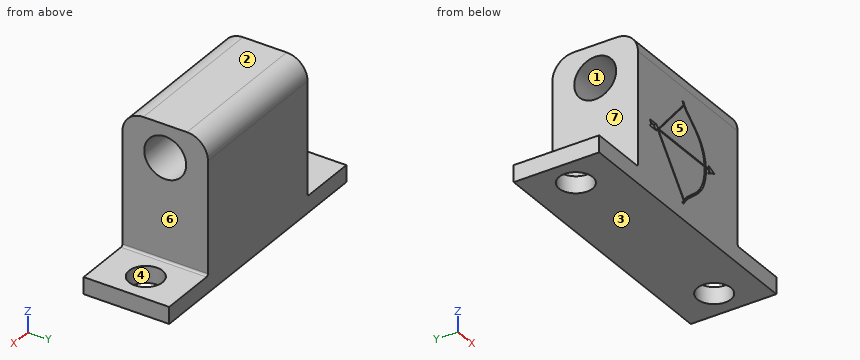
Autodesk Fusion 360 part; units mm, degrees
sketch "Sketch1" plane through (0, 0, 0) normal (0, 0, 1) x (1, 0, 0)
  line L0 (0, 0) -> (32, 0)
  line L1 (32, 0) -> (32, 10.2)
  line L2 (32, 10.2) -> (0, 10.2)
  line L3 (0, 10.2) -> (0, 0)
  dimension "d1" = 32
  dimension "d2" = 10.2
extrude "Extrude1" add sketch "Sketch1" along normal blind 2
sketch "Sketch2" plane through (0, 0, 2) normal (0, 0, 1) x (-1, 0, 0)
  line L0 (0, -10.2) -> (0, 0)
  line L1 (0, 0) -> (-32, 0)
  line L2 (-32, 0) -> (-32, -10.2)
  line L3 (-32, -10.2) -> (0, -10.2)
  line L4 (-7, -10.2) -> (-25, -10.2)
  line L5 (-25, -10.2) -> (-25, 0)
  line L6 (-25, 0) -> (-7, 0)
  line L7 (-7, 0) -> (-7, -10.2)
  circle A0 centre (-3.5, -5.1) radius 2
  circle A1 centre (-28.5, -5.1) radius 2
  dimension "d5" = 7
  dimension "d6" = 7
  dimension "d7" = 5.1
  dimension "d8" = 3.5
  dimension "d9" = 4
  dimension "d10" = 3.5
  dimension "d11" = 5.1
  dimension "d12" = 4
extrude "Extrude2" cut sketch "Sketch2" against normal blind 2.1 contours A0 | A1
extrude "Extrude3" add sketch "Sketch2" along normal blind 16 contours L1 L3 L4 L5 L6 L7
sketch "Sketch3" plane through (25, 0, 0) normal (1, 0, 0) x (0, 1, 0)
  line L0 (0, 2) -> (10.2, 2)
  line L1 (10.2, 2) -> (10.2, 18)
  line L2 (10.2, 18) -> (0, 18)
  line L3 (0, 18) -> (0, 2)
  circle A0 centre (5.1, 14.1) radius 2.5
  dimension "d17" = 3.9
  dimension "d18" = 5.1
  dimension "d19" = 5
extrude "Extrude4" cut sketch "Sketch3" against normal blind 20 contours A0
fillet "Fillet1" radius 2.5 2 edges at (16, 0, 18) (16, 10.2, 18)
fillet "Fillet2" radius 0.25 2 edges at (25, 5.1, 2) (7, 5.1, 2)
sketch "Sketch4" plane through (0, 0, 0) normal (0, -1, 0) x (1, 0, 0)
  line L0 (25, 15.5) -> (7, 15.5)
  line L1 (7, 15.5) -> (7, 2.25)
  arc A0 (6.75, 2) -> (7, 2.25) centre (6.75, 2.25) ccw
  line L2 (6.75, 2) -> (0, 2)
  line L3 (0, 2) -> (0, 0)
  line L4 (0, 0) -> (32, 0)
  line L5 (32, 0) -> (32, 2)
  line L6 (32, 2) -> (25.25, 2)
  arc A1 (25, 2.25) -> (25.25, 2) centre (25.25, 2.25) ccw
  line L7 (25, 2.25) -> (25, 15.5)
  line L8 (15.0115, 13.8918) -> (15.2499, 13.8388)
  line L9 (15.0115, 1.9217) -> (15.2499, 1.8688)
  line L10 (15.2499, 2.3085) -> (10.5625, 8.1981)
  line L11 (10.6841, 8.3354) -> (15.2499, 13.4918)
  line L12 (10.817, 8.3354) -> (15.3124, 13.4128)
  line L13 (15.3132, 2.3954) -> (10.6954, 8.1981)
  spline S0 degree 5 poles (15.0115, 13.8918) (15.0366, 13.8331) (15.0755, 13.7537) (15.1214, 13.6739) (15.1743, 13.5935) (15.2341, 13.5126) (15.2499, 13.4918) knots 0 0 0 0 0 0 0.04 0.053771 0.053771 0.053771 0.053771 0.053771 0.053771
  line L14 (15.2177, 13.5342) -> (15.2821, 13.4495)
  spline S1 degree 5 poles (15.2499, 2.3085) (15.2476, 2.3054) (15.194, 2.2294) (15.1434, 2.1527) (15.0959, 2.0753) (15.0514, 1.9972) (15.0115, 1.9217) knots 0.958261 0.958261 0.958261 0.958261 0.958261 0.958261 0.96 1 1 1 1 1 1
  line L15 (15.2777, 2.3478) -> (15.2221, 2.2693)
  line L16 (19.8903, 8.1981) -> (19.6849, 7.759)
  line L17 (19.6849, 7.759) -> (20.8035, 8.2887)
  line L18 (20.8035, 8.2887) -> (19.6849, 8.7197)
  line L19 (19.6849, 8.7197) -> (19.8674, 8.3354)
  spline S2 degree 5 poles (15.2499, 13.8388) (15.275, 13.7801) (15.3328, 13.6621) (15.4428, 13.4833) (15.636, 13.2415) (15.9534, 12.9319) (16.3409, 12.6103) (16.7857, 12.2676) (17.2659, 11.8886) (17.7534, 11.4561) (18.2174, 10.9546) (18.6276, 10.3741) (18.9469, 9.734) (19.126, 9.1768) (19.2132, 8.7476) (19.2502, 8.4653) (19.263, 8.3354) knots 0 0 0 0 0 0 0.04 0.08 0.12 0.16 0.2 0.24 0.28 0.32 0.36 0.4 0.44 0.473865 0.473865 0.473865 0.473865 0.473865 0.473865
  line L20 (19.1848, 9.1287) -> (19.3411, 7.542)
  spline S3 degree 5 poles (19.2746, 8.1981) (19.2853, 8.0482) (19.2958, 7.7438) (19.2774, 7.2862) (19.1846, 6.69) (18.9625, 5.9984) (18.6463, 5.3801) (18.2572, 4.8452) (17.8198, 4.3863) (17.3603, 3.9873) (16.904, 3.6275) (16.4734, 3.2862) (16.0845, 2.9471) (15.7463, 2.6009) (15.5197, 2.3146) (15.375, 2.094) (15.2897, 1.9443) (15.2499, 1.8688) knots 0.481014 0.481014 0.481014 0.481014 0.481014 0.481014 0.52 0.56 0.6 0.64 0.68 0.72 0.76 0.8 0.84 0.88 0.92 0.96 1 1 1 1 1 1
  line L21 (19.2097, 9.1087) -> (19.3396, 7.2875)
  spline S4 degree 5 poles (15.3124, 13.4128) (15.332, 13.3889) (15.4036, 13.3041) (15.5393, 13.1573) (15.762, 12.9459) (16.1025, 12.6633) (16.5474, 12.3206) (17.0276, 11.9416) (17.515, 11.5091) (17.979, 11.0075) (18.3892, 10.427) (18.7131, 9.7778) (18.894, 9.2098) (18.9811, 8.7693) (19.0172, 8.476) (19.0296, 8.3354) knots 0.064218 0.064218 0.064218 0.064218 0.064218 0.064218 0.08 0.12 0.16 0.2 0.24 0.28 0.32 0.36 0.4 0.44 0.476625 0.476625 0.476625 0.476625 0.476625 0.476625
  line L22 (14.9219, 13.8881) -> (15.7028, 12.9376)
  line L23 (18.9651, 9.0672) -> (19.094, 7.6035)
  spline S5 degree 5 poles (19.0398, 8.1981) (19.0483, 8.0587) (19.0561, 7.765) (19.0358, 7.3185) (18.9432, 6.7334) (18.7242, 6.0513) (18.408, 5.433) (18.0189, 4.8982) (17.5814, 4.4393) (17.1219, 4.0403) (16.6657, 3.6805) (16.235, 3.3392) (15.8681, 3.0192) (15.6141, 2.7622) (15.4485, 2.5703) (15.3521, 2.4471) (15.3132, 2.3954) knots 0.483768 0.483768 0.483768 0.483768 0.483768 0.483768 0.52 0.56 0.6 0.64 0.68 0.72 0.76 0.8 0.84 0.88 0.92 0.948678 0.948678 0.948678 0.948678 0.948678 0.948678
  line L24 (18.989, 9.0312) -> (19.0905, 7.3649)
  line L25 (15.7537, 2.9821) -> (14.8727, 1.8087)
  line L26 (10.6954, 8.1981) -> (19.0398, 8.1981)
  line L27 (19.2746, 8.1981) -> (19.8903, 8.1981)
  line L28 (19.263, 8.3354) -> (19.8674, 8.3354)
  line L29 (10.6725, 8.3354) -> (10.3002, 8.665)
  line L30 (10.3002, 8.665) -> (9.1473, 8.665)
  line L31 (9.1473, 8.665) -> (9.409, 8.2777)
  line L32 (9.409, 8.2777) -> (9.1615, 7.917)
  line L33 (9.1615, 7.917) -> (10.3, 7.917)
  line L34 (10.3, 7.917) -> (10.5625, 8.1981)
  line L35 (10.6725, 8.3354) -> (10.6841, 8.3354)
  line L36 (10.817, 8.3354) -> (19.0296, 8.3354)
  point P0 (16.3357, 12.6206)
  point P1 (16.627, 3.4048)
  point P2 (18.7456, 10.1048)
  point P3 (18.825, 5.7617)
  point P4 (18.5867, 5.8147)
  point P5 (18.5072, 10.1578)
  point P6 (16.0973, 12.6736)
  point P7 (16.3886, 3.4577)
extrude "Extrude5" cut sketch "Sketch4" against normal blind 0.3 contours L8 L9 S0 L14 S1 L15 S2 L20 S3 L21 S4 L22 L23 S5 L24 L25 | L16 L17 L18 L19 L20 L21 L27 L28 | L10 L11 L12 L13 L14 L15 L22 L23 L24 L25 L26 L29 L30 L31 L32 L33 L34 L35 L36
sketch "Sketch5" plane through (0, 0, 18) normal (0, 0, 1) x (-1, 0, 0)
  line L0 (-25, -7.7) -> (-7, -7.7)
  line L1 (-7, -7.7) -> (-7, -2.5)
  line L2 (-7, -2.5) -> (-25, -2.5)
  line L3 (-25, -2.5) -> (-25, -7.7)
  line L4 (-7, -10.2) -> (-25, -10.2)
  line L5 (-25, -10.2) -> (-25, 0)
  line L6 (-25, 0) -> (-7, 0)
  line L7 (-7, 0) -> (-7, -10.2)
  point P0 (-7, -10.2)
  point P1 (-25, 0)
sketch "Sketch6" plane through (16, 5.1, 19.1) normal (0, 0, 1) x (1, 0, 0)
  line L0 (-9, 5.1) -> (9, 5.1)
  line L1 (9, 5.1) -> (9, -5.1)
  line L2 (9, -5.1) -> (-9, -5.1)
  line L3 (-9, -5.1) -> (-9, 5.1)
  point P0 (-9, 5.1)
  point P1 (9, -5.1)
extrude "Extrude6" add 1 faces at (19, 4.2333, 18) along direction (0, 0, 1) blind 1.1
sketch "Sketch7" plane through (16, 0, 18.55) normal (0, -1, 0) x (1, 0, 0)
  line L0 (-9, -3.05) -> (9, -3.05)
  line L1 (9, -3.05) -> (9, 0.55)
  line L2 (9, 0.55) -> (-9, 0.55)
  line L3 (-9, 0.55) -> (-9, -3.05)
  point P0 (-9, -3.05)
  point P1 (9, 0.55)
sketch "Sketch8" plane through (0, 0, 0) normal (0, -1, 0) x (1, 0, 0)
  line L0 (9.409, 8.2777) -> (9.1473, 8.665)
  line L1 (9.1473, 8.665) -> (10.3002, 8.665)
  line L2 (10.3002, 8.665) -> (10.6725, 8.3354)
  line L3 (10.6725, 8.3354) -> (10.6841, 8.3354)
  line L4 (10.6841, 8.3354) -> (15.2499, 13.4918)
  spline S0 degree 5 poles (15.2499, 13.4918) (15.2341, 13.5126) (15.1743, 13.5935) (15.1214, 13.6739) (15.0755, 13.7537) (15.0366, 13.8331) (15.0115, 13.8918) knots -0.053771 -0.053771 -0.053771 -0.053771 -0.053771 -0.053771 -0.04 0 0 0 0 0 0
  line L5 (15.0115, 13.8918) -> (15.2499, 13.8388)
  spline S1 degree 5 poles (15.2499, 13.8388) (15.275, 13.7801) (15.3328, 13.6621) (15.4428, 13.4833) (15.636, 13.2415) (15.9534, 12.9319) (16.3409, 12.6103) (16.7857, 12.2676) (17.2659, 11.8886) (17.7534, 11.4561) (18.2174, 10.9546) (18.6276, 10.3741) (18.9469, 9.734) (19.126, 9.1768) (19.2132, 8.7476) (19.2502, 8.4653) (19.263, 8.3354) knots 0 0 0 0 0 0 0.04 0.08 0.12 0.16 0.2 0.24 0.28 0.32 0.36 0.4 0.44 0.473865 0.473865 0.473865 0.473865 0.473865 0.473865
  line L6 (19.263, 8.3354) -> (19.8674, 8.3354)
  line L7 (19.8674, 8.3354) -> (19.6849, 8.7197)
  line L8 (19.6849, 8.7197) -> (20.8035, 8.2887)
  line L9 (20.8035, 8.2887) -> (19.6849, 7.759)
  line L10 (19.6849, 7.759) -> (19.8903, 8.1981)
  line L11 (19.8903, 8.1981) -> (19.2746, 8.1981)
  spline S2 degree 5 poles (19.2746, 8.1981) (19.2853, 8.0482) (19.2958, 7.7438) (19.2774, 7.2862) (19.1846, 6.69) (18.9625, 5.9984) (18.6463, 5.3801) (18.2572, 4.8452) (17.8198, 4.3863) (17.3603, 3.9873) (16.904, 3.6275) (16.4734, 3.2862) (16.0845, 2.9471) (15.7463, 2.6009) (15.5197, 2.3146) (15.375, 2.094) (15.2897, 1.9443) (15.2499, 1.8688) knots 0.481014 0.481014 0.481014 0.481014 0.481014 0.481014 0.52 0.56 0.6 0.64 0.68 0.72 0.76 0.8 0.84 0.88 0.92 0.96 1 1 1 1 1 1
  line L12 (15.2499, 1.8688) -> (15.0115, 1.9217)
  spline S3 degree 5 poles (15.0115, 1.9217) (15.0514, 1.9972) (15.0959, 2.0753) (15.1434, 2.1527) (15.194, 2.2294) (15.2476, 2.3054) (15.2499, 2.3085) knots -1 -1 -1 -1 -1 -1 -0.96 -0.958261 -0.958261 -0.958261 -0.958261 -0.958261 -0.958261
  line L13 (15.2499, 2.3085) -> (10.5625, 8.1981)
  line L14 (10.5625, 8.1981) -> (10.3, 7.917)
  line L15 (10.3, 7.917) -> (9.1615, 7.917)
  line L16 (9.1615, 7.917) -> (9.409, 8.2777)
  line L17 (25, 15.5) -> (7, 15.5)
  line L18 (7, 15.5) -> (7, 2.25)
  arc A0 (6.75, 2) -> (7, 2.25) centre (6.75, 2.25) ccw
  line L19 (6.75, 2) -> (0, 2)
  line L20 (0, 2) -> (0, 0)
  line L21 (0, 0) -> (32, 0)
  line L22 (32, 0) -> (32, 2)
  line L23 (32, 2) -> (25.25, 2)
  arc A1 (25, 2.25) -> (25.25, 2) centre (25.25, 2.25) ccw
  line L24 (25, 2.25) -> (25, 15.5)
  line L25 (7, 15.5) -> (25, 15.5)
  line L26 (25, 15.5) -> (25, 19.1)
  line L27 (25, 19.1) -> (7, 19.1)
  line L28 (7, 19.1) -> (7, 15.5)
  point P0 (25, 19.1)
sketch "Sketch9" plane through (0, 0, 0) normal (0, -1, 0) x (1, 0, 0)
sketch "Sketch10" plane through (25, 0, 0) normal (1, 0, 0) x (0, 1, 0)
  line L0 (0, 2.25) -> (10.2, 2.25)
  line L1 (10.2, 2.25) -> (10.2, 15.5)
  arc A0 (10.2, 15.5) -> (7.7, 18) centre (7.7, 15.5) ccw
  line L2 (7.7, 18) -> (7.7, 19.1)
  line L3 (7.7, 19.1) -> (2.5, 19.1)
  line L4 (2.5, 19.1) -> (2.5, 18)
  arc A1 (2.5, 18) -> (0, 15.5) centre (2.5, 15.5) ccw
  line L5 (0, 15.5) -> (0, 2.25)
  circle A2 centre (5.1, 14.1) radius 2.5
  line L6 (0, 19.1) -> (10.2, 19.1)
  line L7 (10.2, 19.1) -> (10.2, 10)
  line L8 (10.2, 10) -> (0, 10)
  line L9 (0, 10) -> (0, 19.1)
  line L10 (10.2, 2) -> (10.2, 18)
  point P0 (0, 19.1)
extrude "Extrude7" cut 1 faces at (19, 4.2333, 19.1) along direction (0, 0, -1) blind 1.1
Could you check a few things on this model? Use its own coordinates, in mm. Face numbers are marked on the shaded views. A direction names the side the tool comes from. Give positions to 0.01 mm unless a question says otherwise; leave off trailing zeros. Loops run counter-clockwise (first coordinate to the right, second up) from the corner with the lowest first, then second, coordinate; pieces in that order, holes last. Notation, with made-up numbers: (7, 47) - (47, 47) arc R18 cw to (47, 75) - close; hole circle Ø7 at (65.5, 32). An arc over 180 degrees is marked (long way). Use one line per item in the form item = value.
1. I want a section at B-B (y = 5.1). Please give me the cut outline in (x, z).
Response values:
outline = (0, 0) - (1.5, 0) - (1.5, 2) - (0, 2) - close; (5.5, 0) - (26.5, 0) - (26.5, 2) - (25.25, 2) arc R0.25 cw to (25, 2.25) - (25, 11.6) - (7, 11.6) - (7, 2.25) arc R0.25 cw to (6.75, 2) - (5.5, 2) - close; (7, 16.6) - (25, 16.6) - (25, 18) - (7, 18) - close; (30.5, 0) - (32, 0) - (32, 2) - (30.5, 2) - close
2. I'm going to push flat-ended pins straight in: pin 1 Ø2 at (y, z) = (3, 14.5) entering from -X; pin 2 Ø3 at (y, z) = (7.5, 8.5) entering from +X; pin 3 Ø4.5 at (x, y) = (28.5, 5.1) entering from +Z. Where does each tip first touch, or does it pass through?
Response values:
pin_1 = 7
pin_2 = 25
pin_3 = 2
3. I want a section at A-A (x = 3.5). Please give me the cut outline in (y, z), and give its area (3 significant figures).
Response values:
outline = (0, 0) - (3.1, 0) - (3.1, 2) - (0, 2) - close; (7.1, 0) - (10.2, 0) - (10.2, 2) - (7.1, 2) - close
area = 12.4 mm²
4. I need wall thicknesses on probe 1 along Y at (x, z) = (28.5, 0.9); probe 2 along Z at (x, y) = (18, 5.1); probe 3 along Z at (x, y) = (26.5, 4.75). Which ranges of each line are inside material? Lowest first, please.
Response values:
probe_1 = 0 to 3.1, 7.1 to 10.2
probe_2 = 0 to 11.6, 16.6 to 18
probe_3 = 0 to 2
5. On a 3-axis mill with a long thin cutter (end or side, diameter ignored), from which of +Z, -Z, +X, -X, +Y, -Y can I reach the whole of each face in a straight line? I mean the marked faces 5, 6 and 7. Say none if no direction works.
Response values:
face_5 = +Z, -Z, +X, -X, -Y
face_6 = +Z, +X, +Y, -Y
face_7 = +Z, -X, +Y, -Y
6. Thinking about a two-plate mould opening in Z: for the marked faces 1, 2, 3 and 4, which applies, released by +Z, released by -Z, zero draft, split by the parting line, or undercut?
Response values:
face_1 = undercut
face_2 = released by +Z
face_3 = released by -Z
face_4 = zero draft
7. I want a section at C-C (x = 24.5). Please give me the cut outline in (y, z), and give its area (3 significant figures).
Response values:
outline = (0, 0) - (10.2, 0) - (10.2, 15.5) arc R2.5 ccw to (7.7, 18) - (2.5, 18) arc R2.5 ccw to (0, 15.5) - close; hole circle Ø5 at (5.1, 14.1)
area = 161 mm²
8. I want a section at D-D (y = 8.75). Please give me the cut outline in (x, z).
Response values:
outline = (0, 0) - (32, 0) - (32, 2) - (25.25, 2) arc R0.25 cw to (25, 2.25) - (25, 17.77) - (7, 17.77) - (7, 2.25) arc R0.25 cw to (6.75, 2) - (0, 2) - close
